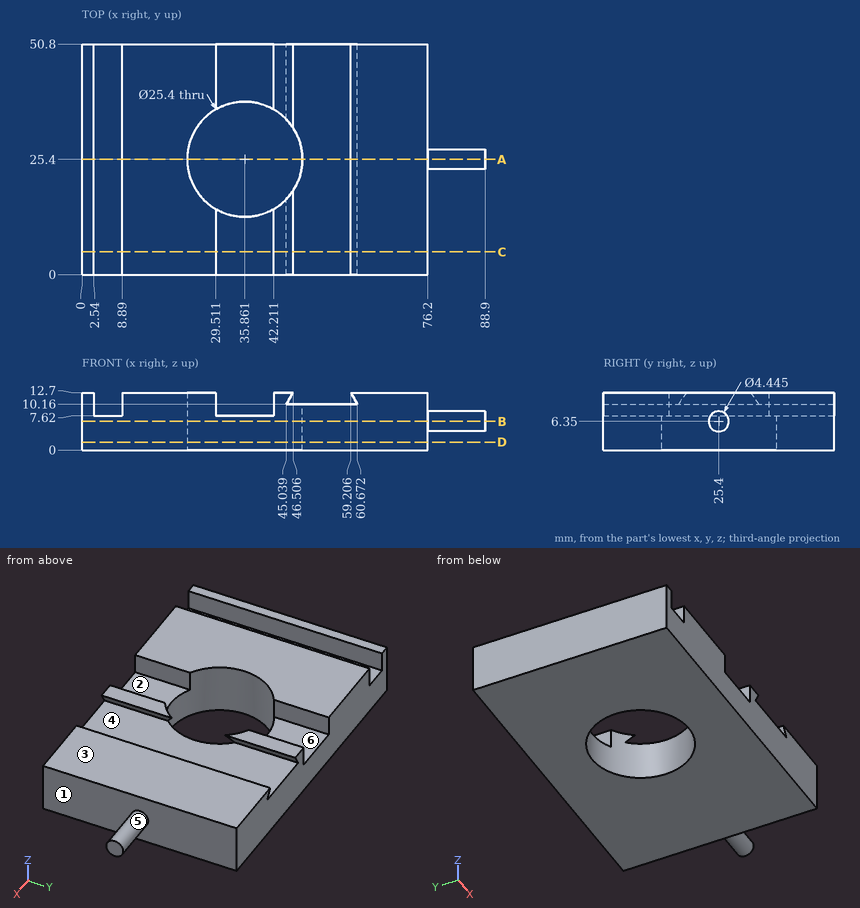
Here's the drawing with two shaded views (mm, measured from the low corner). I have some questions. A direction names the side the tool comes from. Give positions to 0.01 mm unless a question says otherwise; leave off trailing zeros. Loops run counter-clockwise (first coordinate to the right, second up) from the corner with the lowest first, then second, coordinate; pieces in that order, holes last. Notation, with made-up numbers: (10.25, 16.25) -> (65.25, 16.25) arc R27 cw to (65.25, 47.25) -> close; hole circle Ø8 at (81.5, -19). An arc over 180 degrees is marked (long way). Answer as a JSON object with one key per item and string values. Group by question number.
Item 1: Imagine slicing it at A-A on y = 25.4. Write out the boundary of the cut face in (x, z) (1 decimal).
Item 2: Imagine slicing it at C-C on y = 5. Write out the boundary of the cut face in (x, z) (1 decimal), then the cut area to 3 significant figures.
Item 3: I need wall thicknesses on L1, parallel to X at y = 25.4, z = 8.25; L2, parallel to X at y = 37.5, z = 8; L3, parallel to X at y = 25.4, z = 3.25. Which ranges of each line are inside material? Lowest first, please.
Item 4: Will these pins go through, and if not, where does the flat tip stop? pin 1 (5.5 mm diameter, centred on y = 43.5, z = 10.5, fed in from +X); pin 2 (4 mm diameter, centred on x = 38, z = 10, fed in from +Y) (3 decimals); pin 3 (6 mm diameter, centred on x = 53.5, y = 24, fed in from +Z); pin 4 (4 mm diameter, centred on x = 34.5, y = 10, fed in from +Z).
Item 5: Imagine slicing it at B-B on z = 6.35. Write out the boundary of the cut face in (x, y).
Item 6: On a 3-axis mill with a long thin cutter (end or side, diameter ignored), from which of +Z, -Z, +X, -X, +Y, -Y can I reach the whole of each face in a straight line? I mean the marked faces 4, 5 and 6. Say none if no direction works.
Item 7: Imagine slicing it at D-D on z = 1.75. Write out the boundary of the cut face in (x, y), then the cut area to 3 significant figures.
Item 8: Thinking about a two-plate mould opening in X: for the marked faces 1, 2 and 3, which applies, pulls with the +X half, pulls with the -X half, needs draft (parallel to the pull), parting line crosses it, or undercut?
Answer list:
{
 "1": {"outline": "(0, 0) -> (23.2, 0) -> (23.2, 12.7) -> (8.9, 12.7) -> (8.9, 7.6) -> (2.5, 7.6) -> (2.5, 12.7) -> (0, 12.7) -> close; (48.6, 0) -> (76.2, 0) -> (76.2, 4.1) -> (88.9, 4.1) -> (88.9, 8.6) -> (76.2, 8.6) -> (76.2, 12.7) -> (59.2, 12.7) -> (60.7, 10.2) -> (48.6, 10.2) -> close"},
 "2": {"outline": "(0, 0) -> (76.2, 0) -> (76.2, 12.7) -> (59.2, 12.7) -> (60.7, 10.2) -> (45, 10.2) -> (46.5, 12.7) -> (42.2, 12.7) -> (42.2, 7.6) -> (29.5, 7.6) -> (29.5, 12.7) -> (8.9, 12.7) -> (8.9, 7.6) -> (2.5, 7.6) -> (2.5, 12.7) -> (0, 12.7) -> close", "area": "835 mm2"},
 "3": {"L1": "x = 0 to 2.54, 8.89 to 23.16, 48.56 to 88.9", "L2": "x = 0 to 2.54, 8.89 to 29.51, 42.21 to 76.2", "L3": "x = 0 to 23.16, 48.56 to 76.2"},
 "4": {"pin 1": "stops at x = 76.2", "pin 2": "passes through", "pin 3": "stops at z = 10.16", "pin 4": "stops at z = 7.62"},
 "5": {"outline": "(0, 0) -> (76.2, 0) -> (76.2, 23.18) -> (88.9, 23.18) -> (88.9, 27.62) -> (76.2, 27.62) -> (76.2, 50.8) -> (0, 50.8) -> close; hole circle Ø25.4 at (35.86, 25.4)"},
 "6": {"face 4": "+Y, -Y", "face 5": "+X", "face 6": "+Z, +Y, -Y"},
 "7": {"outline": "(0, 0) -> (76.2, 0) -> (76.2, 50.8) -> (0, 50.8) -> close; hole circle Ø25.4 at (35.86, 25.4)", "area": "3,360 mm2"},
 "8": {"face 1": "pulls with the +X half", "face 2": "undercut", "face 3": "needs draft"}
}
